from build123d import *

# Parameters (mm, degrees)
CHAMFER1_SIZE      = 0.5
CUT_EXTRUDE1_START = -3.000000119
CUT_EXTRUDE1_DEPTH = 3.000000119
FILLET2_R          = 0.25


with BuildPart() as part:
    # Sketch1 → Revolve1 (revolve)
    with BuildSketch(Plane(origin=(0, 0, 0), x_dir=(0, 0, -1), z_dir=(1, 0, 0)), mode=Mode.PRIVATE) as revolve1_sk:
        Polygon((0, 5), (-6, 5), (-6, 0), (130, 0), (130, 3), (0, 3), align=None)
    revolve(revolve1_sk.sketch.rotate(Axis((0, 0, 6), (0, 0, -1)), 180), axis=Axis((0, 0, 6), (0, 0, -1)))

    # Sketch7 → Cut-Revolve2 (revolve, cut)
    with BuildSketch(Plane(origin=(0, 0, 0), x_dir=(0, 0, -1), z_dir=(1, 0, 0)), mode=Mode.PRIVATE) as cut_revolve2_sk:
        Polygon((-6, 0), (-6, 2.5), (-3, 2.5), (-1.556624327, 0), align=None)
    revolve(cut_revolve2_sk.sketch.rotate(Axis((0, 0, 6), (0, 0, -1)), 90), axis=Axis((0, 0, 6), (0, 0, -1)), mode=Mode.SUBTRACT)

    # Chamfer1
    chamfer1_edges = [part.edges().sort_by_distance(p)[0] for p in [
        (0, 3, -130),
        (0, 5, 6),
    ]]
    chamfer(chamfer1_edges, length=CHAMFER1_SIZE)

    # Cut-Extrude1: read off the stored shape, not the designer's step
    # Cut-Extrude1 outline → Cut-Extrude1 (cut)
    with BuildSketch(Plane.XY.offset(6).offset(CUT_EXTRUDE1_START)):
        with BuildLine():
            Line((2.5, 0), (2.5, 1.443375673))
            Line((2.5, 1.443375673), (1.249999979, 2.165063522))
            ThreePointArc((1.249999979, 2.165063522), (2.165063503, 1.250000011), (2.5, 0))
        make_face()
        with BuildLine():
            ThreePointArc((-1.250000002, 2.165063508), (-1.4e-08, 2.5), (1.249999979, 2.165063522))
            Line((1.249999979, 2.165063522), (0, 2.886751346))
            Line((0, 2.886751346), (-1.250000002, 2.165063508))
        make_face()
        with BuildLine():
            Line((2.5, -1.443375673), (2.5, 0))
            ThreePointArc((2.5, 0), (2.165063503, -1.250000011), (1.249999979, -2.165063522))
            Line((1.249999979, -2.165063522), (2.5, -1.443375673))
        make_face()
        with BuildLine():
            ThreePointArc((-2.5, 0), (-2.16506351, 1.249999999), (-1.250000002, 2.165063508))
            Line((-1.250000002, 2.165063508), (-2.5, 1.443375673))
            Line((-2.5, 1.443375673), (-2.5, 0))
        make_face()
        with BuildLine():
            Line((0, -2.886751346), (1.249999979, -2.165063522))
            ThreePointArc((1.249999979, -2.165063522), (-1.4e-08, -2.5), (-1.250000002, -2.165063508))
            Line((-1.250000002, -2.165063508), (0, -2.886751346))
        make_face()
        with BuildLine():
            ThreePointArc((-1.250000002, -2.165063508), (-2.16506351, -1.249999999), (-2.5, 0))
            Line((-2.5, 0), (-2.5, -1.443375673))
            Line((-2.5, -1.443375673), (-1.250000002, -2.165063508))
        make_face()
    extrude(amount=CUT_EXTRUDE1_DEPTH, mode=Mode.SUBTRACT)

    # Cut-Extrude1 2 outline → Cut-Extrude1 2 (revolve)
    with BuildSketch(Plane.XZ):
        Polygon((2.886751353, 3.223290998), (2.499999948, 2.99999997), (2.886751346, 2.999999881), align=None)
    revolve(axis=Axis((0, 0, 0), (0, 0, 1)))

    # Sketch9 → Cut-Revolve3 (revolve, cut)
    with BuildSketch(Plane(origin=(0, 0, 0), x_dir=(0, 0, -1), z_dir=(1, 0, 0))):
        Polygon((-6.5, 3.75277675), (-6.5, 2.5), (-5.776709006, 2.5), align=None)
    revolve(axis=Axis((0, 0, 6), (0, 0, -1)), mode=Mode.SUBTRACT)

    # Fillet2
    fillet2_edges = [part.edges().sort_by_distance(p)[0] for p in [
        (0, 3, 0),
    ]]
    fillet(fillet2_edges, radius=FILLET2_R)


solid = part.part
Geometry check sheet. Reference: the model listing, model coordinates, mm. A direction names the side the tool comes from. Round coordinates to 2 decimals unless told otherwise and drop trailing zeros. Loops run counter-clockwise (first coordinate to the right, second up) from the corner with the lowest first, then second, coordinate; pieces in that order, holes last.
Item 1: Cross-section at A-A on z = -35. Record the boundary of the cut face in (x, y), then the cut area to 3 significant figures.
Item 2: Access from +Z, -Z, +X, -X, +Y, -Y to the whole of each face (thin tool, end or side, straight path). Record for faces 1 (the flat face through (2.5, 0, 4)), 2 (the cylindrical face through (-0.9, -2.86, -63.97)), 3 (the flat face through (0, 0, -130)).
Item 3: Thickness scan on line 1 (X direction, y = 0.25, z = -108); line 2 (Z direction, x = -2, y = -2.5). Record the ranges inside material, lowest first.
Item 4: Gauge pin test, flat ends, axial feed: pin 1 (4 mm diameter, centred on x = 1, z = -111, fed in from -Y); pin 2 (2 mm diameter, centred on x = 1, y = 0, fed in from +Z); pin 3 (3 mm diameter, centred on x = 0.5, z = -20, fed in from +Y). Record the tip position at first contact, or that the pin passes through.
Item 5: Mould release check, pull along Y, two halves, no side actions. Record for faces 4 (the flat face through (-2.5, 0, 4)), 5 (the flat face through (3.3, 1, 0)), 6 (the cylindrical face through (0, 5, 3)): pulls with the +Y half, pulls with the -Y half, needs draft (parallel to the pull), parting line crosses it, or undercut.
Answer sheet:
1. outline: circle Ø6 at (0, 0)
1. area: 28.3 mm2
2. face 1: +Z
2. face 2: -Z
2. face 3: -Z, +X, -X, +Y, -Y
3. line 1: x = -2.99 to 2.99
3. line 2: z = 0 to 6
4. pin 1: stops at y = -3
4. pin 2: stops at z = 2.71
4. pin 3: stops at y = 3
5. face 4: undercut
5. face 5: needs draft
5. face 6: parting line crosses it
